```python
from build123d import *

# Parameters (mm, degrees)
SKETCH1_W           = 44.362146026
SKETCH1_H           = 10
BOSS_EXTRUDE1_DEPTH = 18
SKETCH2_R           = 1.6
CUT_EXTRUDE1_DEPTH  = 27
CUT_EXTRUDE2_START  = -17.925297
SKETCH3_R           = 3.05
CUT_EXTRUDE2_DEPTH  = 12.925297
FILLET1_R           = 3


with BuildPart() as part:
    # Sketch1 → Boss-Extrude1 (new body)
    with BuildSketch(Plane.XY):
        with BuildLine():
            Line((-29.953929645, -23), (-37.509998667, -23))
            ThreePointArc((-37.509998667, -23), (-35.812927639, -25.562359318), (-33.941125497, -28))
            Line((-33.941125497, -28), (-22.181073013, -28))
            Line((-22.181073013, -28), (-22.181073013, -23))
            Line((-22.181073013, -23), (-29.953929645, -23))
        make_face()
        with BuildLine():
            Line((-37.509998667, -23), (-43.266615306, -23))
            ThreePointArc((-43.266615306, -23), (0, -49), (43.266615306, -23))
            Line((43.266615306, -23), (37.509998667, -23))
            ThreePointArc((37.509998667, -23), (35.812927639, -25.562359318), (33.941125497, -28))
            ThreePointArc((33.941125497, -28), (28.503075122, -33.519765939), (22.181073013, -38))
            ThreePointArc((22.181073013, -38), (0, -44), (-22.181073013, -38))
            ThreePointArc((-22.181073013, -38), (-28.503075122, -33.519765939), (-33.941125497, -28))
            ThreePointArc((-33.941125497, -28), (-35.812927639, -25.562359318), (-37.509998667, -23))
        make_face()
        with BuildLine():
            Line((-22.181073013, -28), (-33.941125497, -28))
            ThreePointArc((-33.941125497, -28), (-28.503075122, -33.519765939), (-22.181073013, -38))
            Line((-22.181073013, -38), (-22.181073013, -28))
        make_face()
        with BuildLine():
            ThreePointArc((22.181073013, -38), (28.503075122, -33.519765939), (33.941125497, -28))
            Line((33.941125497, -28), (22.181073013, -28))
            Line((22.181073013, -28), (22.181073013, -38))
        make_face()
        with BuildLine():
            ThreePointArc((33.941125497, -28), (35.812927639, -25.562359318), (37.509998667, -23))
            Line((37.509998667, -23), (22.181073013, -23))
            Line((22.181073013, -23), (22.181073013, -28))
            Line((22.181073013, -28), (33.941125497, -28))
        make_face()
        with Locations((0, -33)):
            Rectangle(SKETCH1_W, SKETCH1_H)
        with BuildLine():
            Line((22.181073013, -38), (-22.181073013, -38))
            ThreePointArc((-22.181073013, -38), (0, -44), (22.181073013, -38))
        make_face()
    extrude(amount=BOSS_EXTRUDE1_DEPTH)

    # Sketch2 → Cut-Extrude1 (cut, through all)
    with BuildSketch(Plane(origin=(0, -23, 0), x_dir=(1, 0, 0), z_dir=(0, 1, 0))):
        with Locations((-29.996615306, -9)):
            Circle(SKETCH2_R)
    cut_extrude1 = extrude(amount=-CUT_EXTRUDE1_DEPTH, mode=Mode.SUBTRACT)

    # Sketch3 → Cut-Extrude2 (cut)
    with BuildSketch(Plane(origin=(0, -23, 0), x_dir=(1, 0, 0), z_dir=(0, 1, 0)).offset(CUT_EXTRUDE2_START)):
        with Locations((-29.996615306, -9)):
            Circle(SKETCH3_R)
    cut_extrude2 = extrude(amount=CUT_EXTRUDE2_DEPTH, mode=Mode.SUBTRACT)

    # Mirror1: Cut-Extrude1, Cut-Extrude2 across plane
    add(cut_extrude1.mirror(Plane(origin=(0, 0, 0), x_dir=(0, 0, 1), z_dir=(1, 0, 0))), mode=Mode.SUBTRACT)
    add(cut_extrude2.mirror(Plane(origin=(0, 0, 0), x_dir=(0, 0, 1), z_dir=(1, 0, 0))), mode=Mode.SUBTRACT)

    # Fillet1
    fillet1_edges = [part.edges().sort_by_distance(p)[0] for p in [
        (0, -28, 18),
        (0, -28, 0),
        (22.181073013, -25.5, 0),
        (22.181073013, -23, 9),
        (-22.181073013, -23, 9),
        (-22.181073013, -25.5, 18),
        (-32.723844159, -23, 18),
        (0, -49, 18),
        (32.723844159, -23, 18),
        (22.181073013, -25.5, 18),
        (32.723844159, -23, 0),
        (0, -49, 0),
        (-32.723844159, -23, 0),
        (-22.181073013, -25.5, 0),
    ]]
    fillet(fillet1_edges, radius=FILLET1_R)


solid = part.part
```
Could you check a few things on this model? Use its own coordinates, in mm. A direction names the side the tool comes from. Coordinates: 2 decimals unless noted, no trailing zeros. Order: outer loops, then holes, each group sorted by start corner. A loop starts at its lowest first (then second) coordinate and runs counter-clockwise, first axis right, second up. Notation, with made-up numbers: M 87.5,63 L 106.5,63 A8 cw 106.5,72 Z; hole C 0.5,4.25 d9. An arc over 180 degrees is marked long. Use a Markdown table: item, result. Add a question column.
Q1. I want a section at C-C on y = -30.25. Give the number of separate pieces and of enclosed holes in the cut face, then the cut area to 3 significant figures.
Q2. Which directions (+Z, -Z, +X, -X, +Y, -Y) give clear straight access to the entire face, cutting with the end or side of a thin tool? Please do faces 1 (the cylindrical face through (-23.433, -27.909, 0.562)), 2 (the cylindrical face through (27.18, -33.12, 10.17)), 3 (the flat face through (22.181, -27, 9)).
Q3. I want a section at B-B on z = 9. List the corners of the cut face in (x, y) for me, then the cut area to 3 significant figures.
Q4. If I drill on L1, parallel to X at y = -33, z = 9; L2, parallel to X at y = -35, z = 9; L3, parallel to X at y = -26.75, z = 9, over which ranges is the centre line in solid material (lowest first)?
Q5. I'm going to push flat-ended pins straight in: pin 1 (2 mm diameter, centred on y = -26.5, z = 11.5, fed in from +X); pin 2 (3.5 mm diameter, centred on x = 0, z = 9, fed in from +Y); pin 3 (1.8 mm diameter, centred on x = 29.5, z = 10.5, fed in from -Y); pin 4 (2.5 mm diameter, centred on x = 30, z = 9, fed in from -Y). Where does each tip first touch, or does it pass through?
Q6. I want a section at A-A on z = 4. List the corners of the cut face in (x, y) for me, then the cut area to 3 significant figures.
Checked values:
| question | item | result |
|---|---|---|
| 1 | separate pieces | 1 |
| 1 | enclosed holes | 2 |
| 1 | area | 1,310 mm² |
| 2 | face 1 | -Z, +Y |
| 2 | face 2 | -Y |
| 2 | face 3 | +Z, -Z, +Y |
| 3 | outline | M -43.27,-23 A49 ccw -33.05,-36.18 L -33.05,-28 L -31.6,-28 L -31.6,-23 Z; M -28.4,-28 L -26.95,-28 L -26.95,-40.93 A49 ccw 26.95,-40.93 L 26.95,-28 L 28.4,-28 L 28.4,-23 L 25.18,-23 A3 ccw 22.18,-26 L 22.18,-28 L -22.18,-28 L -22.18,-26 A3 ccw -25.18,-23 L -28.4,-23 Z; M 31.6,-28 L 33.05,-28 L 33.05,-36.18 A49 ccw 43.27,-23 L 31.6,-23 Z |
| 3 | area | 1,220 mm² |
| 4 | L1 | -36.22 to -33.05, -26.95 to 26.95, 33.05 to 36.22 |
| 4 | L2 | -34.29 to -33.05, -26.95 to 26.95, 33.05 to 34.29 |
| 4 | L3 | -41.05 to -31.6, -28.4 to -22.18, 22.18 to 28.4, 31.6 to 41.05 |
| 5 | pin 1 | x = 41.84 |
| 5 | pin 2 | y = -28 |
| 5 | pin 3 | y = -28 |
| 5 | pin 4 | through |
| 6 | outline | M -43.27,-23 A49 ccw 43.27,-23 L 25.18,-23 A3 ccw 22.18,-26 L 22.18,-28 L -22.18,-28 L -22.18,-26 A3 ccw -25.18,-23 Z |
| 6 | area | 1,380 mm² |
